Verification items for the finished model (mm, model axes). Face numbers are marked on the shaded views. A direction names the side the tool comes from. Round coordinates to 2 decimals unless told otherwise and drop trailing zeros. Loops run counter-clockwise (first coordinate to the right, second up) from the corner with the lowest first, then second, coordinate; pieces in that order, holes last. Notation, with made-up numbers: (56.25, 60) - (88.25, 60) arc R32 ccw to (88.25, 89) - close; hole circle Ø4 at (29.5, 62). An arc over 180 degrees is marked (long way). Use a Markdown table: item, result. Add a question column.
```python
from build123d import *

# Parameters (mm, degrees)
SKETCH1_W           = 82
SKETCH1_H           = 102
BOSS_EXTRUDE1_DEPTH = 45
FILLET1_R           = 15
FILLET2_SIZE        = 10
SKETCH2_W           = 1.935509438
SKETCH2_H           = 108.039568053
CUT_EXTRUDE1_DEPTH  = 25
CUT_EXTRUDE2_DEPTH  = 25
SKETCH4_W           = 64.944344057
SKETCH4_H           = 15.809351463
CUT_EXTRUDE3_DEPTH  = 2
CUT_EXTRUDE4_DEPTH  = 8
SKETCH6_W           = 60.105213435
SKETCH6_H           = 24.98512856
CUT_EXTRUDE5_DEPTH  = 8
SKETCH7_R           = 1.5
CUT_EXTRUDE6_DEPTH  = 8


with BuildPart() as part:
    # Sketch1 → Boss-Extrude1 (new body)
    with BuildSketch(Plane.XY):
        with Locations((-4.71634799, 11.800448269)):
            Rectangle(SKETCH1_W, SKETCH1_H)
    extrude(amount=BOSS_EXTRUDE1_DEPTH)

    # Fillet1
    fillet1_edges = [part.edges().sort_by_distance(p)[0] for p in [
        (-4.71634799, -39.199551731, 45),
    ]]
    fillet(fillet1_edges, radius=FILLET1_R)

    # Fillet2
    # a fillet whose section is not a circle: 10 mm, written as the material it takes off along each edge
    with BuildSketch(Plane(origin=(-70.71634799, 62.800448269, 45), x_dir=(0, -1, 0), z_dir=(1, 0, 0))) as fillet2_piece_1:
        with BuildLine():
            Bezier((FILLET2_SIZE, 0), (0, 0), (0, FILLET2_SIZE), weights=[1, 1, 1])
            Line((0, FILLET2_SIZE), (0, 0))
            Line((0, 0), (FILLET2_SIZE, 0))
        make_face()
    extrude(amount=132, mode=Mode.SUBTRACT)

    # Sketch2 → Cut-Extrude1 (cut)
    with BuildSketch(Plane.XY.offset(45)):
        with Locations((33.920109965, 11.021338758)):
            Rectangle(SKETCH2_W, SKETCH2_H)
    extrude(amount=-CUT_EXTRUDE1_DEPTH, mode=Mode.SUBTRACT)

    # Sketch3 → Cut-Extrude2 (cut)
    with BuildSketch(Plane.XY.offset(45)):
        Polygon((32.952355246, 36.51166629), (28.204087152, 63.475951779), (32.952355246, 63.475951779), align=None)
    extrude(amount=-CUT_EXTRUDE2_DEPTH, mode=Mode.SUBTRACT)

    # Sketch4 → Cut-Extrude3 (cut)
    with BuildSketch(Plane.XY.offset(45)):
        with Locations((-7.429597209, 40.183157287)):
            Rectangle(SKETCH4_W, SKETCH4_H)
    extrude(amount=-CUT_EXTRUDE3_DEPTH, mode=Mode.SUBTRACT)

    # Sketch5 → Cut-Extrude4 (cut)
    with BuildSketch(Plane.XY.offset(45)):
        with BuildLine():
            Line((-37.079623524, -20.597881777), (22.815677351, -20.597881777))
            add(Edge.make_bspline(
                [(-37.079623524, -20.597881777), (-5.102026038, -12.590864718), (22.815677351, -20.597881777)],
                knots=[0, 0, 0, 0.561199211, 0.561199211, 0.561199211], degree=2))
        make_face()
    extrude(amount=-CUT_EXTRUDE4_DEPTH, mode=Mode.SUBTRACT)

    # Sketch6 → Cut-Extrude5 (cut)
    with BuildSketch(Plane.XY.offset(45)):
        with Locations((-7.027016807, -33.090446057)):
            Rectangle(SKETCH6_W, SKETCH6_H)
    extrude(amount=-CUT_EXTRUDE5_DEPTH, mode=Mode.SUBTRACT)

    # Sketch7 → Cut-Extrude6 (cut)
    with BuildSketch(Plane(origin=(0, 0, 0), x_dir=(-1, 0, 0), z_dir=(0, 0, -1))):
        with Locations((-28.78365201, 47.800448269)):
            Circle(SKETCH7_R)
        with Locations((38.21634799, 47.800448269)):
            Circle(SKETCH7_R)
        with Locations((38.21634799, -24.199551731)):
            Circle(SKETCH7_R)
        with Locations((-28.78365201, -24.199551731)):
            Circle(SKETCH7_R)
    extrude(amount=-CUT_EXTRUDE6_DEPTH, mode=Mode.SUBTRACT)


solid = part.part
```
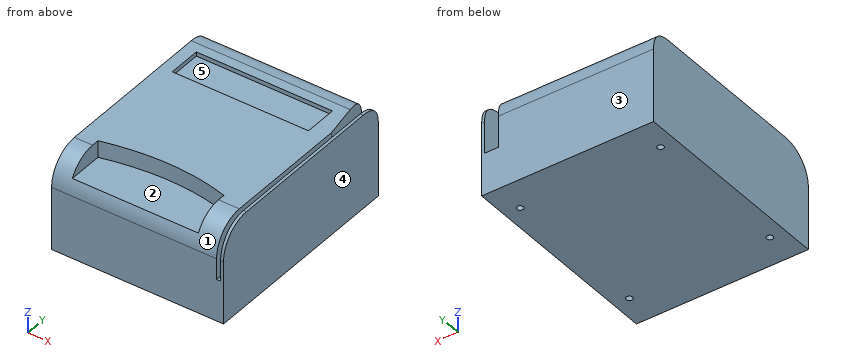
Q1. Section check C-C on y = -27. Record the cut outline in (x, z).
Q2. Go/stop test with flat-tipped pins: pin 1 Ø1.5 at (x, y) = (-1, 32.5) entering from -Z; pin 2 Ø1.6 at (x, z) = (-13.5, 44) entering from -Y; pin 3 Ø5 at (x, y) = (-12, -28.5) entering from +Z; pin 4 Ø2 at (x, z) = (-4, 44) entering from +Y. Record where each tip stops, or that it passes through.
Q3. Section check A-A on z = 23.5. Record the cut outline in (x, y).
Q4. Section check B-B on y = 44. Record the cut outline in (x, z).
Q5. Release check for a two-part mould opening along Y. For the marked faces 3, 4 and 5 record: +Y half, -Y half, draft (parallel to the pull), parting line (faces both ways), or undercut.
Q6. Set-up check for the marked faces 1 and 2: record each of +Z, -Z, +X, -X, +Y, -Y from which the full face is reachable in a straight line by a thin tool's end or side.
Q7. Thickness scan on line 1 along X through (y, z) = (15.5, 21); line 2 along Z through (x, y) = (32, 44); line 3 along X through (y, z) = (46.5, 35.5). Record the ranges inside material, lowest first.
Determined:
| question | item | result |
|---|---|---|
| 1 | outline | (-45.72, 0) - (36.28, 0) - (36.28, 44.74) - (34.89, 44.74) - (34.89, 20) - (32.95, 20) - (32.95, 44.74) - (23.03, 44.74) - (23.03, 37) - (-37.08, 37) - (-37.08, 44.74) - (-45.72, 44.74) - close |
| 2 | pin 1 | stops at z = 0 |
| 2 | pin 2 | stops at y = -16.89 |
| 2 | pin 3 | stops at z = 37 |
| 2 | pin 4 | stops at y = 59.74 |
| 3 | outline | (-45.72, -39.2) - (32.95, -39.2) - (32.95, 36.51) - (28.32, 62.8) - (-45.72, 62.8) - close; (34.89, -39.2) - (36.28, -39.2) - (36.28, 62.8) - (34.89, 62.8) - close |
| 4 | outline | (-45.72, 0) - (36.28, 0) - (36.28, 45) - (34.89, 45) - (34.89, 20) - (31.63, 20) - (31.63, 45) - (25.04, 45) - (25.04, 43) - (-39.9, 43) - (-39.9, 45) - (-45.72, 45) - close |
| 5 | face 3 | +Y half |
| 5 | face 4 | draft |
| 5 | face 5 | undercut |
| 6 | face 1 | +Z, +X, -X, -Y |
| 6 | face 2 | +Z, -Y |
| 7 | line 1 | x = -45.72 to 32.95, 34.89 to 36.28 |
| 7 | line 2 | z = 0 to 20 |
| 7 | line 3 | x = -45.72 to 31.19, 34.89 to 36.28 |
